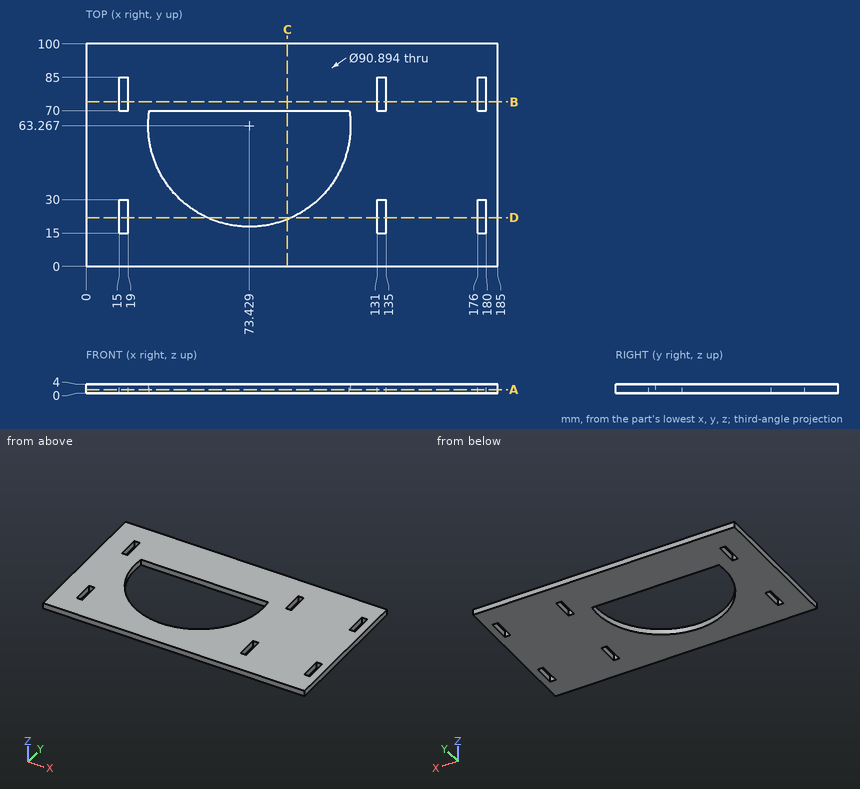
Geometry check sheet. Reference: drawing and pictorial views, mm from the part's lowest x, y, z. Give positions to 0.01 mm unless a question says otherwise; leave off trailing zeros. Loops run counter-clockwise (first coordinate to the right, second up) from the corner with the lowest first, then second, coordinate; pieces in that order, holes last.
1. Section check A-A, the plane z = 1.7. Count the separate pieces of the cut face and the enclosed holes in it, then the cut area to 3 significant figures.
2. Thickness scan on line 1 (X direction, y = 72.5, z = 1.15); line 2 (X direction, y = 33.5, z = 1.7); line 3 (X direction, y = 48, z = 3.6) (1 decimal). Record the ranges inside material, lowest first.
3. Section check D-D, the plane y = 22. Enter the section's corners in (x, z).
4. Section check C-C, the plane x = 90.5. Enter the section's corners in (y, z).
5. Section check B-B, the plane y = 74. Enter the section's corners in (x, z), then the cut area to 3 significant figures.
Geometry says:
1. separate pieces: 1
1. enclosed holes: 7
1. area: 14,300 mm2
2. line 1: x = 0 to 15, 19 to 131, 135 to 176, 180 to 185
2. line 2: x = 0 to 39.09, 107.77 to 185
2. line 3: x = 0 to 30.6, 116.2 to 185
3. outline: (0, 0) - (15, 0) - (15, 4) - (0, 4) - close; (19, 0) - (54.39, 0) - (54.39, 4) - (19, 4) - close; (92.47, 0) - (131, 0) - (131, 4) - (92.47, 4) - close; (135, 0) - (176, 0) - (176, 4) - (135, 4) - close; (180, 0) - (185, 0) - (185, 4) - (180, 4) - close
4. outline: (0, 0) - (21.15, 0) - (21.15, 4) - (0, 4) - close; (70, 0) - (100, 0) - (100, 4) - (70, 4) - close
5. outline: (0, 0) - (15, 0) - (15, 4) - (0, 4) - close; (19, 0) - (131, 0) - (131, 4) - (19, 4) - close; (135, 0) - (176, 0) - (176, 4) - (135, 4) - close; (180, 0) - (185, 0) - (185, 4) - (180, 4) - close
5. area: 692 mm2
